from build123d import *

# Parameters (mm, degrees)
F1_DEPTH = 25


with BuildPart() as f1:
    # F0 (on Top) → F1 (new body)
    with BuildSketch(Plane.XY):
        with BuildLine():
            ThreePointArc((-57.953546, 30.607847), (-57.446882, 29.499646), (-58.416757, 28.761975))
            ThreePointArc((-58.416757, 28.761975), (-58.529898, 27.261975), (-58.416757, 25.761975))
            ThreePointArc((-58.416757, 25.761975), (-57.465205, 25.019706), (-57.953546, 23.916103))
            ThreePointArc((-57.953546, 23.916103), (-57.47113, 22.783765), (-56.853262, 21.719268))
            ThreePointArc((-56.853262, 21.719268), (-55.274335, 21.414336), (-55.196246, 19.808131))
            ThreePointArc((-55.196246, 19.808131), (-53.98712, 18.882314), (-52.651435, 18.150832))
            ThreePointArc((-52.651435, 18.150832), (-51.023986, 18.833197), (-50.029898, 17.375115))
            ThreePointArc((-50.029898, 17.375115), (-48.529898, 17.261975), (-47.029898, 17.375115))
            ThreePointArc((-47.029898, 17.375115), (-46.370381, 18.370345), (-45.196815, 18.150832))
            Line((-45.196815, 18.150832), (-45.051432, 17.88646))
            ThreePointArc((-45.051432, 17.88646), (-43.684454, 18.514308), (-42.42712, 19.3401))
            ThreePointArc((-42.42712, 19.3401), (-42.178457, 21.333884), (-40.206533, 21.719268))
            ThreePointArc((-40.206533, 21.719268), (-39.672157, 22.620808), (-39.235069, 23.573323))
            ThreePointArc((-39.235069, 23.573323), (-39.776693, 24.894231), (-38.643038, 25.761975))
            ThreePointArc((-38.643038, 25.761975), (-38.529898, 27.261975), (-38.643038, 28.761975))
            ThreePointArc((-38.643038, 28.761975), (-39.8333, 29.614407), (-39.235069, 30.950627))
            ThreePointArc((-39.235069, 30.950627), (-39.672157, 31.903142), (-40.206533, 32.804682))
            ThreePointArc((-40.206533, 32.804682), (-42.145818, 33.109806), (-42.280061, 35.068353))
            ThreePointArc((-42.280061, 35.068353), (-43.176683, 35.708459), (-44.138275, 36.246053))
            ThreePointArc((-44.138275, 36.246053), (-45.946858, 35.535483), (-47.029898, 37.148835))
            ThreePointArc((-47.029898, 37.148835), (-48.529898, 37.261975), (-50.029898, 37.148835))
            ThreePointArc((-50.029898, 37.148835), (-50.61582, 36.41435), (-51.46214, 36.822412))
            ThreePointArc((-51.46214, 36.822412), (-51.598865, 36.779403), (-51.734959, 36.734439))
            ThreePointArc((-51.734959, 36.734439), (-52.416275, 36.475881), (-53.076951, 36.168394))
            ThreePointArc((-53.076951, 36.168394), (-53.658255, 35.846842), (-54.216927, 35.487405))
            ThreePointArc((-54.216927, 35.487405), (-54.521365, 33.482235), (-56.536531, 33.25312))
            ThreePointArc((-56.536531, 33.25312), (-57.344831, 31.98394), (-57.953546, 30.607847))
        make_face()
        Polygon((-48.936209, 27.612536), (-48.958612, 27.631866), (-48.914976, 27.631866), (-48.777016, 27.75746), (-48.560186, 27.954854), (-48.532724, 27.979855), (-48.532735, 27.904934), (-48.484508, 27.817237), (-48.317012, 27.512652), (-48.181242, 27.440397), (-48.256187, 27.402044), (-48.529898, 27.261975), (-48.946691, 27.048684), (-48.719861, 27.425874), align=None, mode=Mode.SUBTRACT)
        with BuildLine():
            Line((-31.436215, 37.792423), (-40.206533, 32.804682))
            ThreePointArc((-40.206533, 32.804682), (-39.672157, 31.903142), (-39.235069, 30.950627))
            Line((-39.235069, 30.950627), (-30.186063, 35.487405))
            Line((-30.186063, 35.487405), (-31.436215, 37.792423))
        make_face()
        with BuildLine():
            Line((39.470102, 65.261975), (-80.529898, 65.261975))
            ThreePointArc((-80.529898, 65.261975), (-87.600965, 62.333043), (-90.529898, 55.261975))
            Line((-90.529898, 55.261975), (-90.529898, 1.261975))
            ThreePointArc((-90.529898, 1.261975), (-87.600965, -5.809093), (-80.529898, -8.738025))
            Line((-80.529898, -8.738025), (39.470102, -8.738025))
            ThreePointArc((39.470102, -8.738025), (46.54117, -5.809093), (49.470102, 1.261975))
            Line((49.470102, 1.261975), (49.470102, 55.261975))
            ThreePointArc((49.470102, 55.261975), (46.54117, 62.333043), (39.470102, 65.261975))
        make_face()
        with BuildLine():
            Line((-68.473568, 28.761975), (-58.416757, 28.761975))
            ThreePointArc((-58.416757, 28.761975), (-57.446882, 29.499646), (-57.953546, 30.607847))
            Line((-57.953546, 30.607847), (-66.917042, 35.130452))
            ThreePointArc((-66.917042, 35.130452), (-66.497391, 36.046573), (-66.032131, 36.940396))
            ThreePointArc((-66.032131, 36.940396), (-65.904858, 37.167061), (-65.774651, 37.392053))
            ThreePointArc((-65.774651, 37.392053), (-65.655057, 37.592944), (-65.533122, 37.792423))
            Line((-65.533122, 37.792423), (-56.536531, 33.25312))
            ThreePointArc((-56.536531, 33.25312), (-54.521365, 33.482235), (-54.216927, 35.487405))
            Line((-54.216927, 35.487405), (-59.048139, 44.272754))
            ThreePointArc((-59.048139, 44.272754), (-57.871931, 44.946047), (-56.652824, 45.538136))
            Line((-56.652824, 45.538136), (-51.734959, 36.734439))
            ThreePointArc((-51.734959, 36.734439), (-51.598865, 36.779403), (-51.46214, 36.822412))
            ThreePointArc((-51.46214, 36.822412), (-50.61582, 36.41435), (-50.029898, 37.148835))
            Line((-50.029898, 37.148835), (-50.029898, 47.205646))
            ThreePointArc((-50.029898, 47.205646), (-48.529898, 47.261975), (-47.029898, 47.205646))
            Line((-47.029898, 47.205646), (-47.029898, 37.148835))
            ThreePointArc((-47.029898, 37.148835), (-45.946858, 35.535483), (-44.138275, 36.246053))
            Line((-44.138275, 36.246053), (-39.168957, 44.936046))
            ThreePointArc((-39.168957, 44.936046), (-38.800059, 44.735677), (-38.435449, 44.527609))
            ThreePointArc((-38.435449, 44.527609), (-37.632597, 44.03245), (-36.853985, 43.499988))
            Line((-36.853985, 43.499988), (-42.280061, 35.068353))
            ThreePointArc((-42.280061, 35.068353), (-42.145818, 33.109806), (-40.206533, 32.804682))
            Line((-40.206533, 32.804682), (-31.436215, 37.792423))
            Line((-31.436215, 37.792423), (-30.186063, 35.487405))
            Line((-30.186063, 35.487405), (-39.235069, 30.950627))
            ThreePointArc((-39.235069, 30.950627), (-39.8333, 29.614407), (-38.643038, 28.761975))
            Line((-38.643038, 28.761975), (-28.586227, 28.761975))
            ThreePointArc((-28.586227, 28.761975), (-28.55178, 28.197294), (-28.533318, 27.631866))
            ThreePointArc((-28.533318, 27.631866), (-28.537899, 26.696301), (-28.586227, 25.761975))
            Line((-28.586227, 25.761975), (-38.643038, 25.761975))
            ThreePointArc((-38.643038, 25.761975), (-39.776693, 24.894231), (-39.235069, 23.573323))
            Line((-39.235069, 23.573323), (-30.165696, 19.3401))
            Line((-30.165696, 19.3401), (-31.436215, 16.645359))
            Line((-31.436215, 16.645359), (-40.206533, 21.312802))
            Line((-40.206533, 21.312802), (-40.492028, 21.312802))
            ThreePointArc((-40.492028, 21.312802), (-40.346756, 21.514262), (-40.206533, 21.719268))
            ThreePointArc((-40.206533, 21.719268), (-42.178457, 21.333884), (-42.42712, 19.3401))
            Line((-42.42712, 19.3401), (-37.579988, 10.525802))
            ThreePointArc((-37.579988, 10.525802), (-38.866042, 9.751695), (-40.206533, 9.076222))
            Line((-40.206533, 9.076222), (-45.051432, 17.88646))
            Line((-45.051432, 17.88646), (-45.196815, 18.150832))
            ThreePointArc((-45.196815, 18.150832), (-46.370381, 18.370345), (-47.029898, 17.375115))
            Line((-47.029898, 17.375115), (-47.029898, 7.318304))
            ThreePointArc((-47.029898, 7.318304), (-48.529898, 7.261975), (-50.029898, 7.318304))
            Line((-50.029898, 7.318304), (-50.029898, 17.375115))
            ThreePointArc((-50.029898, 17.375115), (-51.023986, 18.833197), (-52.651435, 18.150832))
            Line((-52.651435, 18.150832), (-57.354282, 9.313988))
            ThreePointArc((-57.354282, 9.313988), (-58.916154, 10.170291), (-60.395644, 11.16216))
            Line((-60.395644, 11.16216), (-55.196246, 19.808131))
            ThreePointArc((-55.196246, 19.808131), (-55.274335, 21.414336), (-56.853262, 21.719268))
            Line((-56.853262, 21.719268), (-65.774651, 17.131897))
            ThreePointArc((-65.774651, 17.131897), (-66.481765, 18.445487), (-67.088998, 19.808131))
            Line((-67.088998, 19.808131), (-57.953546, 23.916103))
            ThreePointArc((-57.953546, 23.916103), (-57.465205, 25.019706), (-58.416757, 25.761975))
            Line((-58.416757, 25.761975), (-68.473568, 25.761975))
            ThreePointArc((-68.473568, 25.761975), (-68.529898, 27.261975), (-68.473568, 28.761975))
        make_face(mode=Mode.SUBTRACT)
    extrude(amount=F1_DEPTH)


solid = f1.part
Input: part model. Units: mm. Frame: model coordinates. A direction names the side the tool comes from. Give positions to 0.01 mm unless a question says otherwise; leave off trailing zeros. Loops run counter-clockwise (first coordinate to the right, second up) from the corner with the lowest first, then second, coordinate; pieces in that order, holes last. Notation, with made-up numbers: M 52,21 L 90,21 A18 ccw 90,39 Z; hole C 58.25,81 d3. An arc over 180 degrees is marked long. Use CSV: the item, a comma, the result in double quotes.
(1) Section A-A, the plane y = 14.5. Return loops of the section in (x, z).
Outcome:
outline,"M -90.53,0 L -58.39,0 L -58.39,25 L -90.53,25 Z; M -54.59,0 L -50.03,0 L -50.03,25 L -54.59,25 Z; M -47.03,0 L -43.19,0 L -43.19,25 L -47.03,25 Z; M -39.77,0 L 49.47,0 L 49.47,25 L -39.77,25 Z"
(2) Set-up query: faces 4 (the face through (-58.895, 10.157, 12.325)), 5 (the face through (-90.53, 29, 12)). Return all of +Z, -Z, +X, -X, +Y, -Y with unobstructed straight access to the full face (end or side cutting, diameter ignored); none if empty.
Outcome:
face 4,"+Z, -Z"
face 5,"+Z, -Z, -X, +Y, -Y"
(3) Pin query (flat end, axial travel): P1, Ø6, axis at y = 57.5, z = 18.5, coming from the -X side. Return the tip coordinate at first contact, or that it passes through.
Outcome:
P1,"stops at x = -90.53"
(4) Pull-direction query (X, two-part tool) for faces 1 (the face through (-87.523, 62.41, 12.325)), 2 (the face through (-66.473, 18.427, 12.325)), 3 (the face through (-21, -8.738, 12)); classes: pulls with the +X half, pulls with the -X half, needs draft (parallel to the pull), parting line crosses it, or undercut.
Outcome:
face 1,"pulls with the -X half"
face 2,"undercut"
face 3,"needs draft"
(5) Material intervals for L1, parallel to X at y = 30, z = 14.5; L2, parallel to Y at x = -65, z = 4.5; L3, parallel to Y at x = -29, z = 19.25, sorted ascending. Write a range as [from, to].
Outcome:
L1,"x = [-90.53, -57.45], [-39.87, 49.47]"
L2,"y = [-8.74, 17.53], [20.75, 25.76], [28.76, 34.16], [37.52, 65.26]"
L3,"y = [-8.74, 25.76], [28.76, 65.26]"
